Source: three-view drawing plus pictorial views. Frame: mm from the lowest corner of the part. A direction names the side the tool comes from. Give positions to 0.01 mm unless a question says otherwise; leave off trailing zeros. Order: outer loops, then holes, each group sorted by start corner. A loop starts at its lowest first (then second) coordinate and runs counter-clockwise, first axis right, second up. Notation, with made-up numbers: (-22, 13.25) - (-8, 13.25) arc R10 cw to (-8, 20.25) - close; hole circle Ø6 at (53.25, 65). An arc over 180 degrees is marked (long way). Use CSV: the item, a comma, the result in double quotes.
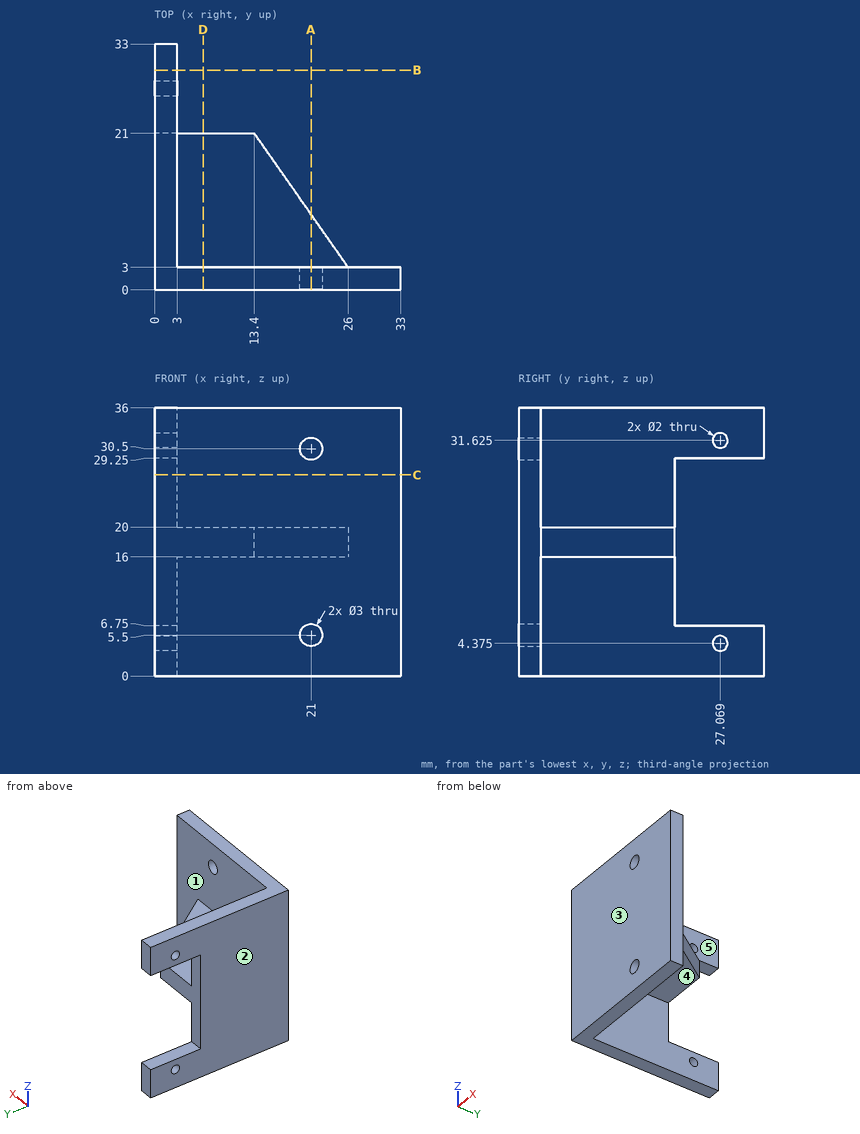
Item 1: Section C-C on z = 27. Return the cut outline in (x, y).
Filled in:
outline,"(0, 0) - (33, 0) - (33, 3) - (3, 3) - (3, 21) - (0, 21) - close"
Item 2: Material intervals for line 1 (Z direction, x = 21, y = 1); line 2 (X direction, y = 2, z = 30.5); line 3 (Y direction, x = 11, z = 13), sorted ascending. Write a range as from..to.
Filled in:
line 1,"z = 0..4, 7..29, 32..36"
line 2,"x = 0..19.5, 22.5..33"
line 3,"y = 0..3"
Item 3: Section A-A on x = 21. Return the cut outline in (y, z).
Filled in:
outline,"(0, 0) - (3, 0) - (3, 4) - (0, 4) - close; (0, 7) - (3, 7) - (3, 16) - (10.14, 16) - (10.14, 20) - (3, 20) - (3, 29) - (0, 29) - close; (0, 32) - (3, 32) - (3, 36) - (0, 36) - close"
Item 4: Set-up query: the marked faces 1, 2, 3, 4 and 5. Return all of +Z, -Z, +X, -X, +Y, -Y with unobstructed straight access to the full face (end or side cutting, diameter ignored); none if empty.
Filled in:
face 1,"+X, +Y"
face 2,"+Z, -Z, -X, +Y, -Y"
face 3,"+Z, -Z, +X, -X, -Y"
face 4,"-Z, +X, +Y"
face 5,"+Z, +X, +Y"
Item 5: First-contact query: pin 1 (13 mm diameter, centred on y = 16, z = 31.5, fed in from +X); pin 2 (10 mm diameter, centred on x = 16, z = 4, fed in from +Y); pin 3 (1.6 mm diameter, centred on y = 27.07, z = 4.38, fed in from -X); pin 4 (14.5 mm diameter, centred on x = 6.5, z = 14, fed in from +Y). Flat tips, straight axial feed; report the tip coordinate or a pass-through.
Filled in:
pin 1,"stops at x = 3"
pin 2,"stops at y = 3"
pin 3,"passes through"
pin 4,"stops at y = 21"
Item 6: Section D-D on x = 6.5. Return the cut outline in (y, z), then the cut area to 3 significant figures.
Filled in:
outline,"(0, 0) - (3, 0) - (3, 16) - (21, 16) - (21, 20) - (3, 20) - (3, 36) - (0, 36) - close"
area,"180 mm2"
Item 7: Section B-B on y = 29.5. Return the cut outline in (x, z), then the cut area to 3 significant figures.
Filled in:
outline,"(0, 0) - (3, 0) - (3, 6.75) - (0, 6.75) - close; (0, 29.25) - (3, 29.25) - (3, 36) - (0, 36) - close"
area,"40.5 mm2"
